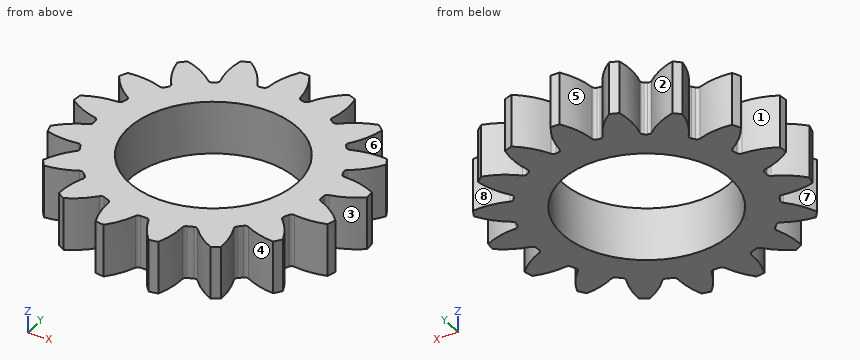
from build123d import *

# Parameters (mm, degrees)
SKETCH_1_R               = 10.875
EXTRUDE_1_DEPTH          = 5
EXTRUDE_2_DEPTH          = 5
FILLET_1_R               = 0.35
PATTERN_CIRCULAR_1_DEPTH = 5
CUT_EXTRUDE_1_REACH      = 22.572
SKETCH_2_R               = 8


# Read off the part's stored shape, not the designer's step: 원형 패턴1
with BuildPart() as part:
    # 스케치1 → 보스-돌출1 (new body)
    with BuildSketch(Plane.XY):
        Circle(SKETCH_1_R)
    extrude(amount=EXTRUDE_1_DEPTH)

    # 스케치1<3> → 보스-돌출2 (add)
    with BuildSketch(Plane.XY):
        with BuildLine():
            ThreePointArc((1.5525, 10.763613183), (1.216970842, 12.576974386), (0.4275, 14.243586057))
            ThreePointArc((0.4275, 14.243586057), (0, 14.25), (-0.4275, 14.243586057))
            ThreePointArc((-0.4275, 14.243586057), (-1.216970842, 12.576974386), (-1.5525, 10.763613183))
            ThreePointArc((-1.5525, 10.763613183), (0, 10.875), (1.5525, 10.763613183))
        make_face()
    extrude(amount=EXTRUDE_2_DEPTH)

    # 필렛1
    fillet_1_edges = [part.edges().sort_by_distance(p)[0] for p in [
        (-1.5525, 10.763613183, 2.5),
        (1.5525, 10.763613183, 2.5),
    ]]
    fillet(fillet_1_edges, radius=FILLET_1_R)

    # 원형 패턴1 outline → 원형 패턴1 (add)
    with BuildSketch(Plane.XY):
        with BuildLine():
            ThreePointArc((2.084837088, 10.673288121), (3.842906104, 10.173381821), (5.492422476, 9.386102511))
            ThreePointArc((5.492422476, 9.386102511), (5.344646109, 9.557145045), (5.332233471, 9.782842475))
            ThreePointArc((5.332233471, 9.782842475), (5.593355494, 11.4564781), (5.452236305, 13.144472855))
            ThreePointArc((5.452236305, 13.144472855), (5.055921411, 13.304884491), (4.654972549, 13.453334479))
            ThreePointArc((4.654972549, 13.453334479), (3.403689946, 12.289385973), (2.465385752, 10.861075951))
            ThreePointArc((2.465385752, 10.861075951), (2.306817266, 10.702930709), (2.084837088, 10.673288121))
        make_face()
        with BuildLine():
            ThreePointArc((5.736195698, 9.2391387), (7.199095251, 8.150990895), (8.459646862, 6.833739823))
            ThreePointArc((8.459646862, 6.833739823), (8.381997736, 7.045900933), (8.450146114, 7.261301773))
            ThreePointArc((8.450146114, 7.261301773), (9.274201483, 8.707038787), (9.740617886, 10.304436202))
            ThreePointArc((9.740617886, 10.304436202), (9.42901262, 10.597181051), (9.108765262, 10.880445977))
            ThreePointArc((9.108765262, 10.880445977), (7.536352291, 10.255192371), (6.155612256, 9.27693802))
            ThreePointArc((6.155612256, 9.27693802), (5.952224819, 9.187903085), (5.736195698, 9.2391387))
        make_face()
        with BuildLine():
            ThreePointArc((8.656847778, 6.582143386), (9.631277253, 5.050160738), (10.337248772, 3.377412148))
            ThreePointArc((10.337248772, 3.377412148), (10.339832595, 3.602419922), (10.478866532, 3.779351375))
            ThreePointArc((10.478866532, 3.779351375), (11.729603042, 4.815098477), (12.713475046, 6.107038785))
            ThreePointArc((12.713475046, 6.107038785), (12.528663426, 6.492580033), (12.332368752, 6.872403399))
            ThreePointArc((12.332368752, 6.872403399), (10.671238348, 6.86130469), (9.057778331, 6.466052652))
            ThreePointArc((9.057778331, 6.466052652), (8.838113972, 6.457792134), (8.656847778, 6.582143386))
        make_face()
        with BuildLine():
            ThreePointArc((10.44566348, 3.025514743), (10.802249116, 1.255802147), (10.861158072, -0.548516485))
            ThreePointArc((10.861158072, -0.548516485), (10.943077602, -0.34062274), (11.134084318, -0.224661311))
            ThreePointArc((11.134084318, -0.224661311), (12.626546762, 0.289328326), (13.969306954, 1.119162384))
            ThreePointArc((13.969306954, 1.119162384), (13.936248813, 1.545430549), (13.890417506, 1.970515105))
            ThreePointArc((13.890417506, 1.970515105), (12.377771936, 2.549980076), (10.773358461, 2.772990553))
            ThreePointArc((10.773358461, 2.772990553), (10.568207288, 2.845653785), (10.44566348, 3.025514743))
        make_face()
        with BuildLine():
            ThreePointArc((10.831434222, -0.972449329), (10.524388312, -2.739137757), (9.931200049, -4.431353133))
            ThreePointArc((9.931200049, -4.431353133), (10.080749628, -4.26807205), (10.298365111, -4.227215102))
            ThreePointArc((10.298365111, -4.227215102), (11.831510548, -4.270865326), (13.338506551, -3.985552654))
            ThreePointArc((13.338506551, -3.985552654), (13.461666574, -3.57612745), (13.572488407, -3.163191729))
            ThreePointArc((13.572488407, -3.163191729), (12.409057254, -2.103647039), (11.041512467, -1.325168872))
            ThreePointArc((11.041512467, -1.325168872), (10.879326869, -1.182845296), (10.831434222, -0.972449329))
        make_face()
        with BuildLine():
            ThreePointArc((9.724818044, -4.867600951), (8.799895988, -6.389636578), (7.638946645, -7.74029193))
            ThreePointArc((7.638946645, -7.74029193), (7.835322049, -7.642919348), (8.051101932, -7.68143897))
            ThreePointArc((8.051101932, -7.68143897), (9.434573038, -8.250170344), (10.906266927, -8.517686277))
            ThreePointArc((10.906266927, -8.517686277), (11.169011671, -8.180399177), (11.421519541, -7.835381548))
            ThreePointArc((11.421519541, -7.835381548), (10.743744256, -6.465085659), (9.78938361, -5.27081353))
            ThreePointArc((9.78938361, -5.27081353), (9.692203368, -5.079599132), (9.724818044, -4.867600951))
        make_face()
        with BuildLine():
            ThreePointArc((7.250855805, -8.104980882), (5.839114845, -9.174440736), (4.272503154, -10.000567074))
            ThreePointArc((4.272503154, -10.000567074), (4.488726043, -9.981391229), (4.674670149, -10.09339498))
            ThreePointArc((4.674670149, -10.09339498), (5.746046713, -11.099844355), (7.00107552, -11.865148727))
            ThreePointArc((7.00107552, -11.865148727), (7.367919852, -11.645552222), (7.728011172, -11.415049228))
            ThreePointArc((7.728011172, -11.415049228), (7.598229184, -9.929070664), (7.162058655, -8.502630716))
            ThreePointArc((7.162058655, -8.502630716), (7.142629708, -8.289552802), (7.250855805, -8.104980882))
        make_face()
        with BuildLine():
            ThreePointArc((3.745858716, -10.209513577), (2.04453627, -10.681081239), (0.289330355, -10.871150489))
            ThreePointArc((0.289330355, -10.871150489), (0.495925275, -10.93192564), (0.627834307, -11.102146342))
            ThreePointArc((0.627834307, -11.102146342), (1.261761796, -12.417365945), (2.150350071, -13.57584665))
            ThreePointArc((2.150350071, -13.57584665), (2.57174963, -13.503598465), (2.990792071, -13.418740812))
            ThreePointArc((2.990792071, -13.418740812), (3.40225572, -12.010026536), (3.516526006, -10.546906395))
            ThreePointArc((3.516526006, -10.546906395), (3.576953157, -10.341342504), (3.745858716, -10.209513577))
        make_face()
        with BuildLine():
            ThreePointArc((-0.289330355, -10.871150489), (-2.04453627, -10.681081239), (-3.745858716, -10.209513577))
            ThreePointArc((-3.745858716, -10.209513577), (-3.576953157, -10.341342504), (-3.516526006, -10.546906395))
            ThreePointArc((-3.516526006, -10.546906395), (-3.40225572, -12.010026536), (-2.990792071, -13.418740812))
            ThreePointArc((-2.990792071, -13.418740812), (-2.57174963, -13.503598465), (-2.150350071, -13.57584665))
            ThreePointArc((-2.150350071, -13.57584665), (-1.261761796, -12.417365945), (-0.627834307, -11.102146342))
            ThreePointArc((-0.627834307, -11.102146342), (-0.495925275, -10.93192564), (-0.289330355, -10.871150489))
        make_face()
        with BuildLine():
            ThreePointArc((-4.272503154, -10.000567074), (-5.839114845, -9.174440736), (-7.250855805, -8.104980882))
            ThreePointArc((-7.250855805, -8.104980882), (-7.142629708, -8.289552802), (-7.162058655, -8.502630716))
            ThreePointArc((-7.162058655, -8.502630716), (-7.598229184, -9.929070664), (-7.728011172, -11.415049228))
            ThreePointArc((-7.728011172, -11.415049228), (-7.367919852, -11.645552222), (-7.00107552, -11.865148727))
            ThreePointArc((-7.00107552, -11.865148727), (-5.746046713, -11.099844355), (-4.674670149, -10.09339498))
            ThreePointArc((-4.674670149, -10.09339498), (-4.488726043, -9.981391229), (-4.272503154, -10.000567074))
        make_face()
        with BuildLine():
            ThreePointArc((-7.638946645, -7.74029193), (-8.799895988, -6.389636578), (-9.724818044, -4.867600951))
            ThreePointArc((-9.724818044, -4.867600951), (-9.692203368, -5.079599132), (-9.78938361, -5.27081353))
            ThreePointArc((-9.78938361, -5.27081353), (-10.743744256, -6.465085659), (-11.421519541, -7.835381548))
            ThreePointArc((-11.421519541, -7.835381548), (-11.169011671, -8.180399177), (-10.906266927, -8.517686277))
            ThreePointArc((-10.906266927, -8.517686277), (-9.434573038, -8.250170344), (-8.051101932, -7.68143897))
            ThreePointArc((-8.051101932, -7.68143897), (-7.835322049, -7.642919348), (-7.638946645, -7.74029193))
        make_face()
        with BuildLine():
            ThreePointArc((-9.931200049, -4.431353133), (-10.524388312, -2.739137757), (-10.831434222, -0.972449329))
            ThreePointArc((-10.831434222, -0.972449329), (-10.879326869, -1.182845296), (-11.041512467, -1.325168872))
            ThreePointArc((-11.041512467, -1.325168872), (-12.409057254, -2.103647039), (-13.572488407, -3.163191729))
            ThreePointArc((-13.572488407, -3.163191729), (-13.461666574, -3.57612745), (-13.338506551, -3.985552654))
            ThreePointArc((-13.338506551, -3.985552654), (-11.831510548, -4.270865326), (-10.298365111, -4.227215102))
            ThreePointArc((-10.298365111, -4.227215102), (-10.080749628, -4.26807205), (-9.931200049, -4.431353133))
        make_face()
        with BuildLine():
            ThreePointArc((-10.861158072, -0.548516485), (-10.802249116, 1.255802147), (-10.44566348, 3.025514743))
            ThreePointArc((-10.44566348, 3.025514743), (-10.568207288, 2.845653785), (-10.773358461, 2.772990553))
            ThreePointArc((-10.773358461, 2.772990553), (-12.377771936, 2.549980076), (-13.890417506, 1.970515105))
            ThreePointArc((-13.890417506, 1.970515105), (-13.936248813, 1.545430549), (-13.969306954, 1.119162384))
            ThreePointArc((-13.969306954, 1.119162384), (-12.626546762, 0.289328326), (-11.134084318, -0.224661311))
            ThreePointArc((-11.134084318, -0.224661311), (-10.943077602, -0.34062274), (-10.861158072, -0.548516485))
        make_face()
        with BuildLine():
            ThreePointArc((-10.337248772, 3.377412148), (-9.631277253, 5.050160738), (-8.656847778, 6.582143386))
            ThreePointArc((-8.656847778, 6.582143386), (-8.838113972, 6.457792134), (-9.057778331, 6.466052652))
            ThreePointArc((-9.057778331, 6.466052652), (-10.671238348, 6.86130469), (-12.332368752, 6.872403399))
            ThreePointArc((-12.332368752, 6.872403399), (-12.528663426, 6.492580033), (-12.713475046, 6.107038785))
            ThreePointArc((-12.713475046, 6.107038785), (-11.729603042, 4.815098477), (-10.478866532, 3.779351375))
            ThreePointArc((-10.478866532, 3.779351375), (-10.339832595, 3.602419922), (-10.337248772, 3.377412148))
        make_face()
        with BuildLine():
            ThreePointArc((-8.459646862, 6.833739823), (-7.199095251, 8.150990895), (-5.736195698, 9.2391387))
            ThreePointArc((-5.736195698, 9.2391387), (-5.952224819, 9.187903085), (-6.155612256, 9.27693802))
            ThreePointArc((-6.155612256, 9.27693802), (-7.536352291, 10.255192371), (-9.108765262, 10.880445977))
            ThreePointArc((-9.108765262, 10.880445977), (-9.42901262, 10.597181051), (-9.740617886, 10.304436202))
            ThreePointArc((-9.740617886, 10.304436202), (-9.274201483, 8.707038787), (-8.450146114, 7.261301773))
            ThreePointArc((-8.450146114, 7.261301773), (-8.381997736, 7.045900933), (-8.459646862, 6.833739823))
        make_face()
        with BuildLine():
            ThreePointArc((-2.465385752, 10.861075951), (-3.403689946, 12.289385973), (-4.654972549, 13.453334479))
            ThreePointArc((-4.654972549, 13.453334479), (-5.055921411, 13.304884491), (-5.452236305, 13.144472855))
            ThreePointArc((-5.452236305, 13.144472855), (-5.593355494, 11.4564781), (-5.332233471, 9.782842475))
            ThreePointArc((-5.332233471, 9.782842475), (-5.344646109, 9.557145045), (-5.492422476, 9.386102511))
            ThreePointArc((-5.492422476, 9.386102511), (-3.842906104, 10.173381821), (-2.084837088, 10.673288121))
            ThreePointArc((-2.084837088, 10.673288121), (-2.306817266, 10.702930709), (-2.465385752, 10.861075951))
        make_face()
    extrude(amount=PATTERN_CIRCULAR_1_DEPTH)

    # 스케치2 → 컷-돌출1 (cut, up to next)
    with BuildSketch(Plane.XY.offset(5), mode=Mode.PRIVATE) as cut_extrude_1_sk1:
        Circle(SKETCH_2_R)
    cut_extrude_1_tool1 = extrude(cut_extrude_1_sk1.sketch, amount=-CUT_EXTRUDE_1_REACH, mode=Mode.PRIVATE) & part.part
    add(cut_extrude_1_tool1.solids().sort_by_distance((0, 0, 5))[0], mode=Mode.SUBTRACT)


solid = part.part
Geometry: final body of the model. Coordinates: model frame, mm. Face numbers are marked on the shaded views. A direction names the side the tool comes from. Give positions to 0.01 mm unless a question says otherwise; leave off trailing zeros. Loops run counter-clockwise (first coordinate to the right, second up) from the corner with the lowest first, then second, coordinate; pieces in that order, holes last. Notation, with made-up numbers: (51.5, -12.75) - (101.5, -12.75) arc R20 ccw to (101.5, -2.75) - close; hole circle Ø4 at (-7.5, 36.25). An arc over 180 degrees is marked (long way). Answer as CSV lines item,"result". Start each with the question number.
1. Reachability of the marked faces 4, 5, 6, 7 and 8 from +Z, -Z, +X, -X, +Y, -Y: full face, straight path, thin tool, end or side. Return the list, or none.
2. Ray query, L1, parallel to Y at x = 0, z = 4.3 (3 decimals); L2, parallel to X at y = -11, z = 0.95; L3, parallel to X at y = 11.5, z = 2.5. Return the intervals inside material, ascending.
3. Draft query along X for the marked faces 1, 2 and 3. Return one class per face: released by +X, released by -X, zero draft, split by the parting line, or undercut.
4. Section B-B, the plane y = -9. Return loops of the section in (x, z).
5. Section A-A, the plane x = -5. Return loops of the section in (y, z) (3 decimals), plus the area to 3 significant figures.
6. Pin query (flat end, axial travel): P1, Ø1, axis at x = 5, z = 1.5, coming from the -Y side; P2, Ø14.5, axis at x = 0, y = 0, coming from the +Z side; P3, Ø1, axis at x = -1, z = 3, coming from the -Y side. Return the tip coordinate at first contact, or that it passes through.
Answers:
1,face 4,"+Z, -Z, -Y"
1,face 5,"+Z, -Z, +Y"
1,face 6,"+Z, -Z, +X"
1,face 7,"+Z, -Z, -X"
1,face 8,"+Z, -Z"
2,L1,"y = -10.875 to -8, 8 to 14.25"
2,L2,"x = -7.72 to -5.62, -3.51 to -0.57, 0.57 to 3.51, 5.62 to 7.72"
2,L3,"x = -5.59 to -2.82, -1.47 to 1.47, 2.82 to 5.59"
3,face 1,"released by -X"
3,face 2,"undercut"
3,face 3,"released by +X"
4,outline,"(-7.35, 0) - (7.35, 0) - (7.35, 5) - (-7.35, 5) - close"
5,outline,"(-10.445, 0) - (-6.245, 0) - (-6.245, 5) - (-10.445, 5) - close; (6.245, 0) - (13.326, 0) - (13.326, 5) - (6.245, 5) - close"
5,area,"56.4 mm2"
6,P1,"stops at y = -10.9"
6,P2,"passes through"
6,P3,"stops at y = -12.78"
